Geometry: see drawing. Coordinates: mm, zero at the bounding-box minimum. Give positions to 0.01 mm unless a question says otherwise; leave off trailing zeros. Loops run counter-clockwise (first coordinate to the right, second up) from the corner with the lowest first, then second, coordinate; pieces in that order, holes last. Notation, with made-up numbers: (-31, 86) - (-1, 86) arc R21 ccw to (-1, 112) - close; hole circle Ø4 at (58.5, 13). An arc over 180 degrees is marked (long way). Use one line per item in the form item = value.
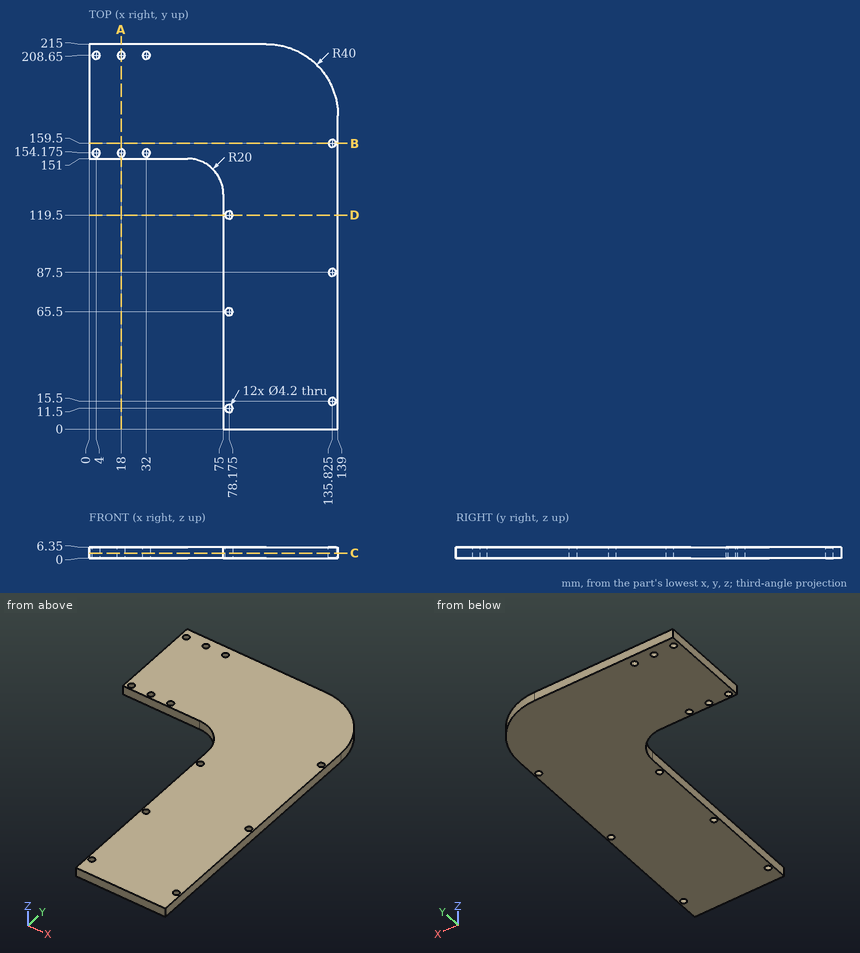
(1) Cut plane D-D (y = 119.5). Return the cut outline in (x, z) (3 decimals).
Solution:
outline = (75, 0) - (76.075, 0) - (76.075, 6.35) - (75, 6.35) - close; (80.275, 0) - (139, 0) - (139, 6.35) - (80.275, 6.35) - close
(2) Cut plane B-B (y = 159.5). Return the cut outline in (x, z) (3 decimals), plus the area to 3 significant figures.
Solution:
outline = (0, 0) - (133.725, 0) - (133.725, 6.35) - (0, 6.35) - close; (137.925, 0) - (139, 0) - (139, 6.35) - (137.925, 6.35) - close
area = 856 mm2
(3) Material intervals for L1, parallel to Y at x = 18, z = 2.5 (3 decimals); L2, parallel to Y at x = 77.5, z = 3.75; L3, parallel to Y at x = 12, z = 3.5, sorted ascending. Write a range as from..to.
Solution:
L1 = 151..152.075, 156.275..206.55, 210.75..215
L2 = 0..9.51, 13.49..63.51, 67.49..117.51, 121.49..215
L3 = 151..215
(4) Pin query (flat end, axial travel): P1, Ø3, axis at y = 22.5, z = 5, coming from the -X side. Return the tip coordinate at first contact, or that it passes through.
Solution:
P1 = 75
(5) Cut plane A-A (x = 18). Return the cut outline in (y, z) (3 decimals), plus the area to 3 significant figures.
Solution:
outline = (151, 0) - (152.075, 0) - (152.075, 6.35) - (151, 6.35) - close; (156.275, 0) - (206.55, 0) - (206.55, 6.35) - (156.275, 6.35) - close; (210.75, 0) - (215, 0) - (215, 6.35) - (210.75, 6.35) - close
area = 353 mm2
(6) Cut plane C-C (z = 3). Give the number of separate pieces and of enclosed holes in the cut face, plus the area to 3 significant figures.
Solution:
separate_pieces = 1
enclosed_holes = 12
area = 18,100 mm2
